from build123d import *

# Parameters (mm, degrees)
SKETCH_1_W          = 100
SKETCH_1_H          = 100
EXTRUDE_1_DEPTH     = 80
SKETCH_2_R          = 5.5
CUT_EXTRUDE_2_DEPTH = 107.77078252
FILLET_1_R          = 10
FILLET_2_R          = 10


with BuildPart() as part:
    # 草图1 → 凸台-拉伸1 (new body)
    with BuildSketch(Plane.XY):
        Rectangle(SKETCH_1_W, SKETCH_1_H)
    extrude(amount=EXTRUDE_1_DEPTH)

    # 草图2 → 切除-拉伸2 (cut, through all)
    with BuildSketch(Plane.XY.offset(80)):
        with Locations((-35, 35)):
            Circle(SKETCH_2_R)
        with Locations((35, 35)):
            Circle(SKETCH_2_R)
        with Locations((-35, -35)):
            Circle(SKETCH_2_R)
        with Locations((35, -35)):
            Circle(SKETCH_2_R)
    extrude(amount=-CUT_EXTRUDE_2_DEPTH, mode=Mode.SUBTRACT)

    # 圆角1
    fillet_1_edges = [part.edges().sort_by_distance(p)[0] for p in [
        (-50, 50, 40),
    ]]
    fillet(fillet_1_edges, radius=FILLET_1_R)

    # 圆角2
    fillet_2_edges = [part.edges().sort_by_distance(p)[0] for p in [
        (50, -50, 40),
        (-50, -50, 40),
        (50, 50, 40),
    ]]
    fillet(fillet_2_edges, radius=FILLET_2_R)


solid = part.part
The model under review builds one solid part; all positions refer to its coordinate system, in mm. Coordinates: 2 decimals unless noted, no trailing zeros. Write each loop counter-clockwise with the first axis right and the second up, starting at its lowest first coordinate (ties: lowest second). Pieces come first, ordered by that corner, then holes. Notation, with made-up numbers: M 73.25,2.25 L 127.25,2.25 A14 cw 127.25,8.25 Z; hole C 49.25,42 d8. An arc over 180 degrees is marked long. Put each result on its own line as item: value.
1) Draft analysis for pull direction X (two halves, no side actions). For faces 1 (the cylindrical face through (-40.495, 35.242, 40.56)), 2 (the cylindrical face through (-40.495, -34.758, 40.56)), 3 (the cylindrical face through (46.99, 47.15, 40.56)), 4 (the flat face through (-1, 1, 80)), state which applies: released by +X, released by -X, zero draft, split by the parting line, or undercut.
Computed:
face 1: undercut
face 2: undercut
face 3: released by +X
face 4: zero draft
2) Wall thickness on probe 1 along Y at (x, z) = (35, 18); probe 2 along X at (y, z) = (-33, 77); probe 3 along X at (y, z) = (-32, 18): over which ranges is each line inside the solid? List them lowest first. Write a range as [from, to].
Computed:
probe 1: y = [-50, -40.5], [-29.5, 29.5], [40.5, 50]
probe 2: x = [-50, -40.12], [-29.88, 29.88], [40.12, 50]
probe 3: x = [-50, -39.61], [-30.39, 30.39], [39.61, 50]
3) Add section A-A on z = 40.5. Give the boundary of the cut face in (x, y), then the cut area to 3 significant figures.
Computed:
outline: M -50,-40 A10 ccw -40,-50 L 40,-50 A10 ccw 50,-40 L 50,40 A10 ccw 40,50 L -40,50 A10 ccw -50,40 Z; hole C -35,-35 d11; hole C -35,35 d11; hole C 35,-35 d11; hole C 35,35 d11
area: 9,530 mm2
4) Add section B-B on x = 35. Give the boundary of the cut face in (y, z).
Computed:
outline: M -50,0 L -40.5,0 L -40.5,80 L -50,80 Z; M -29.5,0 L 29.5,0 L 29.5,80 L -29.5,80 Z; M 40.5,0 L 50,0 L 50,80 L 40.5,80 Z
5) Clearance check with a flat-ended pin moving along its axis: pin 1 Ø9 at (x, y) = (35, -35) entering from -Z. State where the tip first meets the part, or that it passes through.
Computed:
pin 1: passes through
